```python
from build123d import *

# Parameters (mm, degrees)
CUT_EXTRUDE_1_DEPTH = 1.5
FILLET_1_R          = 0.2
CHAMFER_1_SIZE      = 0.2


with BuildPart() as part:
    # 草图1 → 旋转1 (revolve)
    with BuildSketch(Plane.XY, mode=Mode.PRIVATE) as revolve_1_sk:
        Polygon((-8.5, 0), (-8.5, 1.8), (-6.5, 1.8), (-6.5, 1), (8.5, 1), (8.5, 0), align=None)
    revolve(revolve_1_sk.sketch.rotate(Axis((8.5, 0, 0), (-1, 0, 0)), 90), axis=Axis((8.5, 0, 0), (-1, 0, 0)))

    # 草图2 → 切除-拉伸1 (cut)
    with BuildSketch(Plane.ZY.offset(8.5)):
        Polygon((0.866025404, 0), (0.433012702, 0.75), (-0.433012702, 0.75), (-0.866025404, 0), (-0.433012702, -0.75), (0.433012702, -0.75), align=None)
    extrude(amount=-CUT_EXTRUDE_1_DEPTH, mode=Mode.SUBTRACT)

    # 圆角1
    fillet_1_edges = [part.edges().sort_by_distance(p)[0] for p in [
        (-6.5, 0, 1.8),
        (-8.5, 0, 1.8),
    ]]
    fillet(fillet_1_edges, radius=FILLET_1_R)

    # 倒角1
    chamfer_1_edges = [part.edges().sort_by_distance(p)[0] for p in [
        (8.5, 0, 1),
    ]]
    chamfer(chamfer_1_edges, length=CHAMFER_1_SIZE)


solid = part.part
```
Build history of the part. All positions in model axes, mm. A direction names the side the tool comes from. Round coordinates to 2 decimals unless told otherwise and drop trailing zeros. Write each loop counter-clockwise with the first axis right and the second up, starting at its lowest first coordinate (ties: lowest second). Pieces come first, ordered by that corner, then holes. Notation, with made-up numbers: (36.5, 60.5) -> (56.5, 60.5) arc R15 cw to (56.5, 71.5) -> close; hole circle Ø8 at (-3, 74). An arc over 180 degrees is marked (long way). Put each result on its own line as item: value.
Item 1: Flat gauge pins, fed straight in: P1, Ø1.5, axis at x = 0.5, z = 0, coming from the +Y side; P2, Ø2, axis at x = 0, y = 0.5, coming from the +Z side. Where does each tip first touch, or does it go through?
Here are the results:
P1: stops at y = 1
P2: stops at z = 1
Item 2: Slice it at A-A, the plane z = 0. Give the cut face in (x, y).
Here are the results:
outline: (-8.5, -1.6) arc R0.2 ccw to (-8.3, -1.8) -> (-6.7, -1.8) arc R0.2 ccw to (-6.5, -1.6) -> (-6.5, -1) -> (8.3, -1) -> (8.5, -0.8) -> (8.5, 0.8) -> (8.3, 1) -> (-6.5, 1) -> (-6.5, 1.6) arc R0.2 ccw to (-6.7, 1.8) -> (-8.3, 1.8) arc R0.2 ccw to (-8.5, 1.6) -> (-8.5, 0.75) -> (-7, 0.75) -> (-7, -0.75) -> (-8.5, -0.75) -> close
Item 3: Wall check: probe 1 along X at (y, z) = (-0.35, 0.2); probe 2 along Z at (x, y) = (7.25, 0.9); probe 3 along Z at (x, y) = (-5, 0.6). Give the ranges that are in metal, low to high. Write a range as from..to.
Here are the results:
probe 1: x = -7..8.5
probe 2: z = -0.44..0.44
probe 3: z = -0.8..0.8
Item 4: Slice it at B-B, the plane x = -1. Give the cut face in (y, z), plus the area to 3 significant figures.
Here are the results:
outline: circle Ø2 at (0, 0)
area: 3.14 mm^2
Item 5: Tool access for faces 4 (the face through (-8, -0.75, 0)), 5 (the face through (1, 1, 0)), 6 (the face through (8.5, 0, 0)): list every direction of +Z, -Z, +X, -X, +Y, -Y with a clear straight run to the whole face (end or side of a thin tool).
Here are the results:
face 4: -X
face 5: +X
face 6: +Z, -Z, +X, +Y, -Y
Item 6: Two-plate mould, pull along Y, no slides. Class faces 1 (the face through (-7, 0, 0)), 2 (the face through (-8.5, 1, 1)), 3 (the face through (-7.489, -0.541, -1.717)): pulls with the +Y half, pulls with the -Y half, needs draft (parallel to the pull), parting line crosses it, or undercut.
Here are the results:
face 1: undercut
face 2: needs draft
face 3: parting line crosses it
